Here's the drawing with two shaded views (mm, measured from the low corner). I have some questions. A direction names the side the tool comes from. Coordinates: 2 decimals unless noted, no trailing zeros. Loops run counter-clockwise (first coordinate to the right, second up) from the corner with the lowest first, then second, coordinate; pieces in that order, holes last. Notation, with made-up numbers: (36.5, 88) - (71.5, 88) arc R16 cw to (71.5, 101) - close; hole circle Ø6 at (75, 67.5). An arc over 180 degrees is marked (long way). Use a Markdown table: item, result.
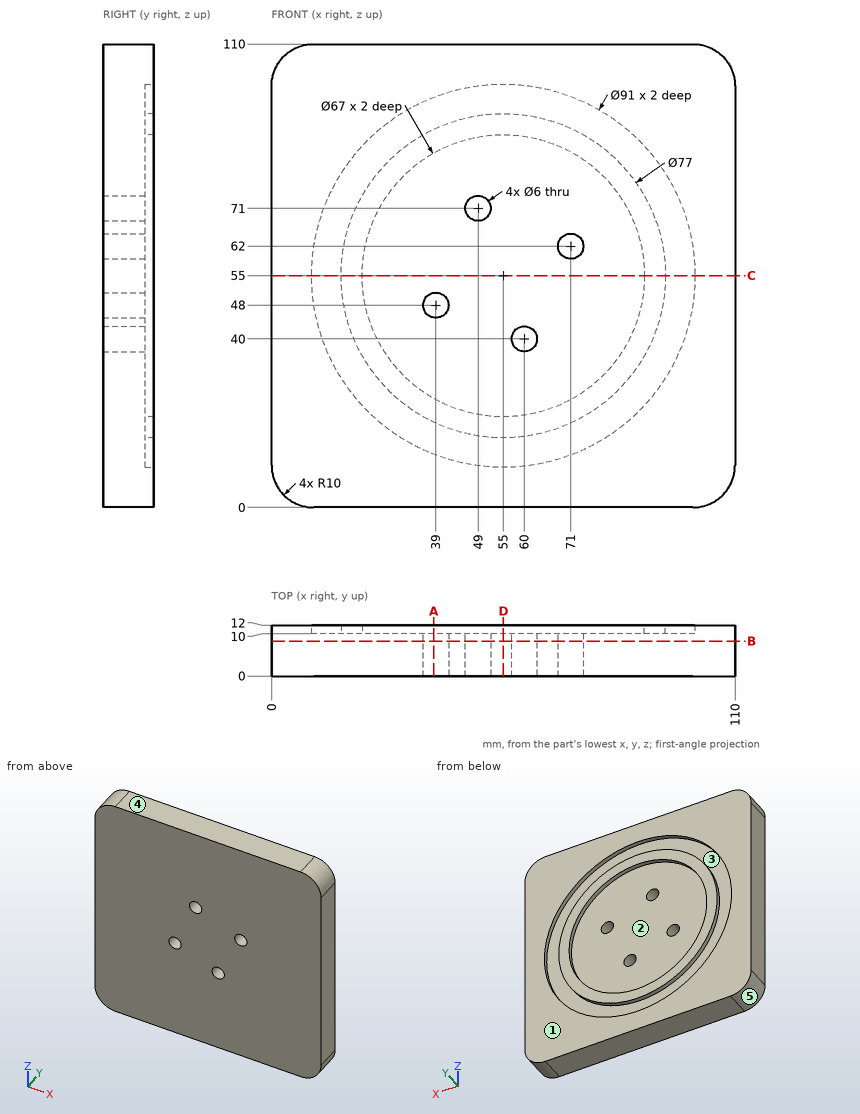
Q1. Which directions (+Z, -Z, +X, -X, +Y, -Y) give clear straight access to the entire face, cutting with the end or side of a thin tool? Please do the marked faces 1 and 2.
Check values:
| item | result |
|---|---|
| face 1 | +Z, -Z, +X, -X, +Y |
| face 2 | +Y |
Q2. Will this pin go through, and if not, where does the flat tip stop? P1, Ø9.5, axis at x = 39, z = 48, coming from the +Y side.
Check values:
| item | result |
|---|---|
| P1 | y = 10 |
Q3. I want a section at A-A, the plane x = 38.5. Write out the boundary of the cut face in (y, z), then the cut area to 3 significant figures.
Check values:
| item | result |
|---|---|
| outline | (0, 0) - (12, 0) - (12, 12.6) - (10, 12.6) - (10, 20.21) - (12, 20.21) - (12, 25.85) - (10, 25.85) - (10, 45.04) - (0, 45.04) - close; (0, 50.96) - (10, 50.96) - (10, 84.15) - (12, 84.15) - (12, 89.79) - (10, 89.79) - (10, 97.4) - (12, 97.4) - (12, 110) - (0, 110) - close |
| area | 1,110 mm^2 |
Q4. Please list where these lines run through material, in increasing order: L1, parallel to Z at x = 55, y = 10.85; L2, parallel to X at y = 11, z = 83.5; L3, parallel to Z at x = 33, y = 11. Write a range as from..to.
Check values:
| item | result |
|---|---|
| L1 | 0..9.5, 16.5..21.5, 88.5..93.5, 100.5..110 |
| L2 | 0..19.53, 29.12..37.39, 72.61..80.88, 90.47..110 |
| L3 | 0..15.17, 23.4..29.74, 80.26..86.6, 94.83..110 |
Q5. If we mould it in two halves opening along X, with no side actions, what happens to the marked faces 3, 4 and 5? For each: pulls with the +X half, pulls with the -X half, needs draft (parallel to the pull), parting line crosses it, or undercut.
Check values:
| item | result |
|---|---|
| face 3 | undercut |
| face 4 | needs draft |
| face 5 | pulls with the -X half |
Q6. I want a section at D-D, the plane x = 55. Write out the boundary of the cut face in (y, z).
Check values:
| item | result |
|---|---|
| outline | (0, 0) - (12, 0) - (12, 9.5) - (10, 9.5) - (10, 16.5) - (12, 16.5) - (12, 21.5) - (10, 21.5) - (10, 88.5) - (12, 88.5) - (12, 93.5) - (10, 93.5) - (10, 100.5) - (12, 100.5) - (12, 110) - (0, 110) - close |
Q7. I want a section at C-C, the plane z = 55. Write out the boundary of the cut face in (x, y).
Check values:
| item | result |
|---|---|
| outline | (0, 0) - (110, 0) - (110, 12) - (100.5, 12) - (100.5, 10) - (93.5, 10) - (93.5, 12) - (88.5, 12) - (88.5, 10) - (21.5, 10) - (21.5, 12) - (16.5, 12) - (16.5, 10) - (9.5, 10) - (9.5, 12) - (0, 12) - close |
Q8. I want a section at B-B, the plane y = 8.25. Write out the boundary of the cut face in (x, z), then the cut area to 3 significant figures.
Check values:
| item | result |
|---|---|
| outline | (0, 10) arc R10 ccw to (10, 0) - (100, 0) arc R10 ccw to (110, 10) - (110, 100) arc R10 ccw to (100, 110) - (10, 110) arc R10 ccw to (0, 100) - close; hole circle Ø6 at (39, 48); hole circle Ø6 at (49, 71); hole circle Ø6 at (60, 40); hole circle Ø6 at (71, 62) |
| area | 11,900 mm^2 |
